Geometry: see drawing. Coordinates: mm, zero at the bounding-box minimum. Give positions to 0.01 mm unless a question says otherwise; leave off trailing zeros. Loops run counter-clockwise (first coordinate to the right, second up) from the corner with the lowest first, then second, coordinate; pieces in that order, holes last. Notation, with made-up numbers: M 44,30.25 L 63,30.25 A11 cw 63,34.25 Z; hole C 73,10 d2. An arc over 180 degrees is marked long. Use a Markdown table: item, result. Add a question column.
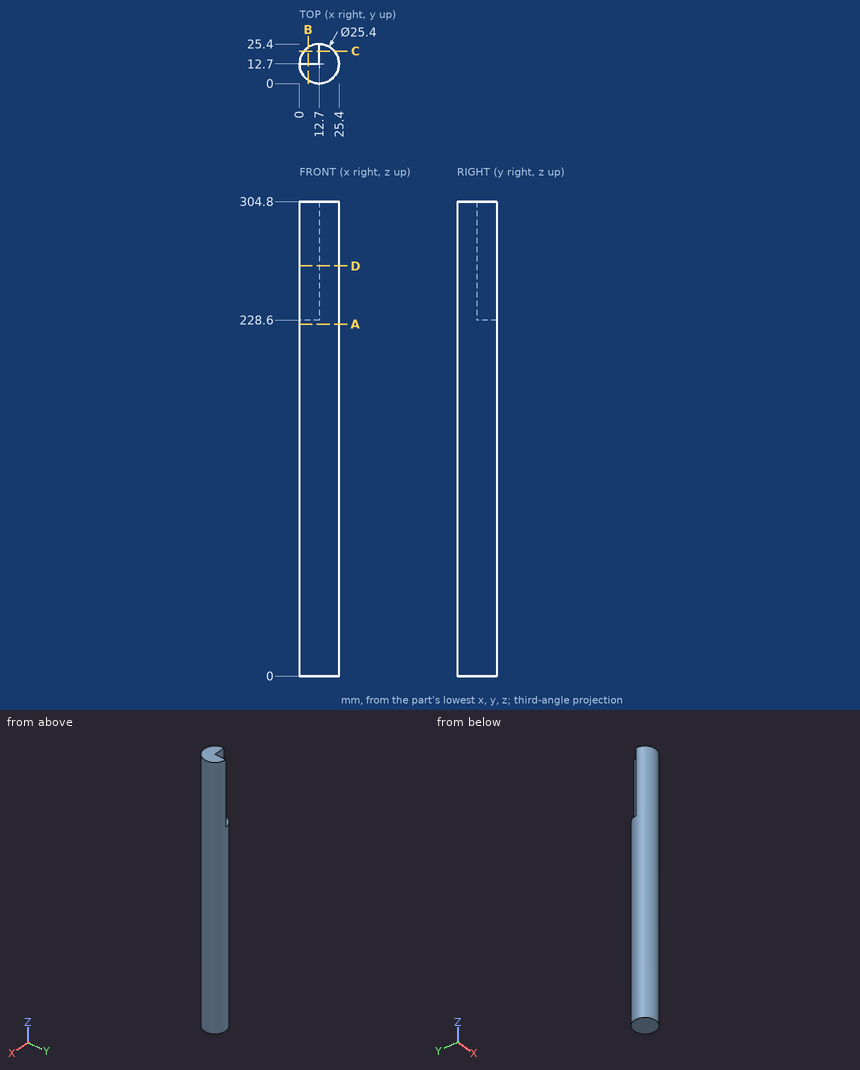
1) Ray query, line 1 (Y direction, x = 13.5, z = 266.5); line 2 (X direction, y = 13, z = 292.5); line 3 (Z direction, x = 2, y = 15.75). Return the intervals inside material, ascending. Write a range as [from, to].
2) Contact query for flat-ended pins moving along their axis: P1, Ø5, axis at x = 20, z = 184, coming from the +Y side; P2, Ø6, axis at x = 5.5, z = 107.5, coming from the +Y side; P3, Ø6.5, axis at y = 20.5, z = 259.5, coming from the -X side. Output: stop coordinate, or through.
3) Section query A-A, the plane z = 226. Return the cut outline in (x, y), and give its area (3 significant figures).
4) Section query D-D, the plane z = 263.5. Return the cut outline in (x, y), and give its area (3 significant figures).
5) Section query B-B, the plane x = 5.5. Return the cut outline in (y, z).
6) Section query C-C, the plane y = 20.75. Return the cut outline in (x, z).
Entries:
| question | item | result |
|---|---|---|
| 1 | line 1 | y = [0.03, 25.37] |
| 1 | line 2 | x = [12.7, 25.4] |
| 1 | line 3 | z = [0, 228.6] |
| 2 | P1 | stops at y = 24.46 |
| 2 | P2 | stops at y = 24.69 |
| 2 | P3 | stops at x = 12.7 |
| 3 | outline | C 12.7,12.7 d25.4 |
| 3 | area | 507 mm² |
| 4 | outline | M 0,12.7 A12.7 ccw long 12.7,25.4 L 12.7,12.7 Z |
| 4 | area | 380 mm² |
| 5 | outline | M 2.24,0 L 23.16,0 L 23.16,228.6 L 12.7,228.6 L 12.7,304.8 L 2.24,304.8 Z |
| 6 | outline | M 2.88,0 L 22.52,0 L 22.52,304.8 L 12.7,304.8 L 12.7,228.6 L 2.88,228.6 Z |
